Part model, mm, in its own coordinate system. A direction names the side the tool comes from. Coordinates: 2 decimals unless noted, no trailing zeros. Write each loop counter-clockwise with the first axis right and the second up, starting at its lowest first coordinate (ties: lowest second). Pieces come first, ordered by that corner, then holes. Notation, with made-up numbers: M 72,-32.5 L 80,-32.5 A17 ccw 80,-27.5 Z; hole C -36,26.25 d7. An arc over 180 degrees is marked long. Use a Markdown table: item, result. Add a question column.
Q1. Pin check, flat tips, straight feed: pin 1 Ø1.5 at (x, y) = (1.5, 13.5) entering from -Z; pin 2 Ø3 at (y, z) = (39.5, 0) entering from -X; pin 3 Ø3 at (x, y) = (1, 42.5) entering from +Z. Stop position of each tip, or through.
Q2. Wall check: L1, parallel to Z at x = 0.05, y = 1.5; L2, parallel to X at y = 41.5, z = 2.05; L3, parallel to Y at x = -0.7, z = -2.6. Give the ranges that are in metal, low to high. Write a range as from..to.
Q3. Mould opens along Z. For faces 1 (the flat face through (-2, 63, 2)), 2 (the flat face through (0, -2, 0)) say: released by +Z, released by -Z, zero draft, split by the parting line, or undercut.
Q4. Tool access for faces 3 (the flat face through (-2, 0, 2)), 4 (the flat face through (0, 65, 0)): list every direction of +Z, -Z, +X, -X, +Y, -Y with a clear straight run to the whole face (end or side of a thin tool).
Q5. Slice it at A-A on y = 11. Write the cut outline in (x, z), then the cut area to 3 significant figures.
Q6. Slice it at B-B on z = 0. Write the cut outline in (x, y).
from build123d import *

# Parameters (mm, degrees)
REVOLVE_1_ANGLE     = 180
CUT_EXTRUDE_1_DEPTH = 1
SKETCH_3_R          = 2.44
EXTRUDE_1_DEPTH     = 31.5


with BuildPart() as part:
    # 草图1 → 旋转1 (revolve)
    with BuildSketch(Plane(origin=(0, 0, 0), x_dir=(1, 0, 0), z_dir=(0, 1, 0))):
        with BuildLine():
            Line((-0.227216636, -2.991383058), (0.227216636, 2.991383058))
            ThreePointArc((0.227216636, 2.991383058), (-2.991383058, 0.227216636), (-0.227216636, -2.991383058))
        make_face()
    revolve(axis=Axis((0.227216636, 0, -2.991383058), (-0.07573887865673318, 0, 0.9971276860361569)), revolution_arc=REVOLVE_1_ANGLE)

    # 草图2 → 切除-拉伸1 (cut)
    with BuildSketch(Plane(origin=(0, -3, 0), x_dir=(-1, 0, 0), z_dir=(0, -1, 0))):
        Polygon((1.161360834, -0.646595492), (1.140648539, 0.68247024), (-0.020712296, 1.329065731), (-1.161360834, 0.646595492), (-1.140648539, -0.68247024), (0.020712296, -1.329065731), align=None)
    extrude(amount=-CUT_EXTRUDE_1_DEPTH, mode=Mode.SUBTRACT)

    # 草图3 → 凸台-拉伸1 (add)
    with BuildSketch(Plane(origin=(0, 0, 0), x_dir=(1, 0, 0), z_dir=(0, 1, 0))):
        Circle(SKETCH_3_R)
    extrude(amount=EXTRUDE_1_DEPTH)

    # 镜向1: part across plane


with BuildPart() as part_1:
    add(part.part)
    add(part.part.mirror(Plane.ZX.offset(31.5)))


solid = part_1.part
Recorded:
| question | item | result |
|---|---|---|
| 1 | pin 1 | z = -2.32 |
| 1 | pin 2 | x = -2.44 |
| 1 | pin 3 | z = 2.44 |
| 2 | L1 | -2.44..2.44 |
| 2 | L2 | -1.32..1.32 |
| 2 | L3 | -1.32..0, 63..64.32 |
| 3 | face 1 | zero draft |
| 3 | face 2 | undercut |
| 4 | face 3 | none |
| 4 | face 4 | +Y |
| 5 | outline | C 0,0 d4.88 |
| 5 | area | 18.7 mm² |
| 6 | outline | M -3,0 A3 ccw -1.15,-2.77 L -1.15,-2 L 1.15,-2 L 1.15,-2.77 A3 ccw 3,0 L 2.44,0 L 2.44,63 L 3,63 A3 ccw 1.15,65.77 L 1.15,65 L -1.15,65 L -1.15,65.77 A3 ccw -3,63 L -2.44,63 L -2.44,0 Z |
